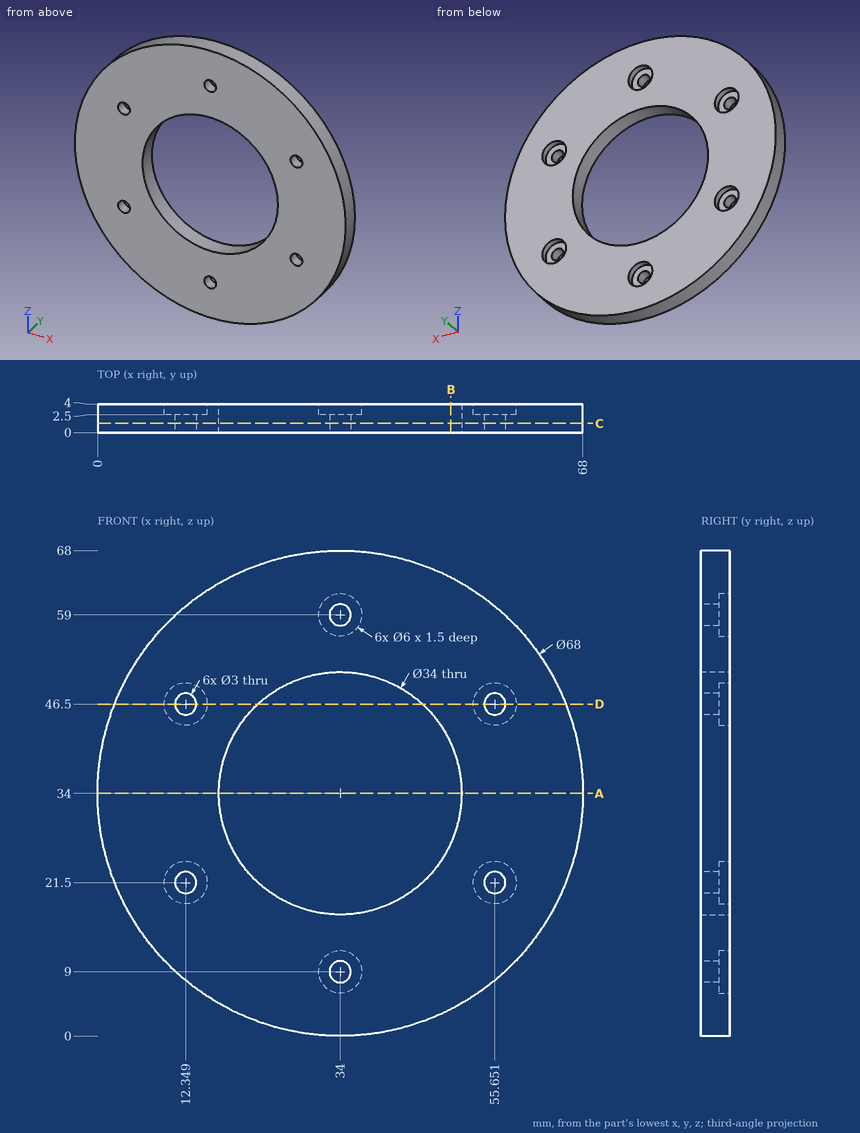
Print and shaded views of the part. All mm, measured from the part's lowest x, y and z. Round coordinates to 2 decimals unless told otherwise and drop trailing zeros. Order: outer loops, then holes, each group sorted by start corner. A loop starts at its lowest first (then second) coordinate and runs counter-clockwise, first axis right, second up.
Q1. Slice it at A-A (z = 34). Write the cut outline in (x, y), and give its area (3 significant figures).
Q2. Slice it at B-B (x = 49.5). Write the cut outline in (y, z).
Q3. Drop flat-ended pins along their axis: pin 1 (1.8 mm diameter, centred on x = 56, z = 45.5, fed in from +Y); pin 2 (1.5 mm diameter, centred on y = 1, z = 11.5, fed in from +X). Give the stop position or say it passes through.
Q4. Slice it at D-D (z = 46.5). Write the cut outline in (x, y), and give its area (3 significant figures).
Q5. Wall check: L1, parallel to X at y = 3.2, z = 46.5; L2, parallel to Z at x = 56.5, y = 1.9 (1 decimal); L3, parallel to Z at x = 11, y = 1.4 (1 decimal). Give the ranges that are in metal, low to high.
Q6. Slice it at C-C (y = 1.3). Write the cut outline in (x, z).
Results below:
1. outline: (0, 0) - (17, 0) - (17, 4) - (0, 4) - close; (51, 0) - (68, 0) - (68, 4) - (51, 4) - close
1. area: 136 mm2
2. outline: (0, 3.74) - (4, 3.74) - (4, 27.02) - (0, 27.02) - close; (0, 40.98) - (4, 40.98) - (4, 64.26) - (0, 64.26) - close
3. pin 1: stops at y = 2.5
3. pin 2: stops at x = 60.13
4. outline: (2.38, 0) - (10.85, 0) - (10.85, 2.5) - (9.35, 2.5) - (9.35, 4) - (2.38, 4) - close; (13.85, 0) - (22.48, 0) - (22.48, 4) - (15.35, 4) - (15.35, 2.5) - (13.85, 2.5) - close; (45.52, 0) - (54.15, 0) - (54.15, 2.5) - (52.65, 2.5) - (52.65, 4) - (45.52, 4) - close; (57.15, 0) - (65.62, 0) - (65.62, 4) - (58.65, 4) - (58.65, 2.5) - (57.15, 2.5) - close
4. area: 128 mm2
5. L1: x = 2.38 to 9.35, 15.35 to 22.48, 45.52 to 52.65, 58.65 to 65.62
5. L2: z = 8.5 to 20.3, 22.7 to 45.3, 47.7 to 59.5
5. L3: z = 9 to 20.8, 22.2 to 45.8, 47.2 to 59
6. outline: circle Ø68 at (34, 34); hole circle Ø3 at (12.35, 21.5); hole circle Ø3 at (12.35, 46.5); hole circle Ø34 at (34, 34); hole circle Ø3 at (34, 9); hole circle Ø3 at (34, 59); hole circle Ø3 at (55.65, 21.5); hole circle Ø3 at (55.65, 46.5)
